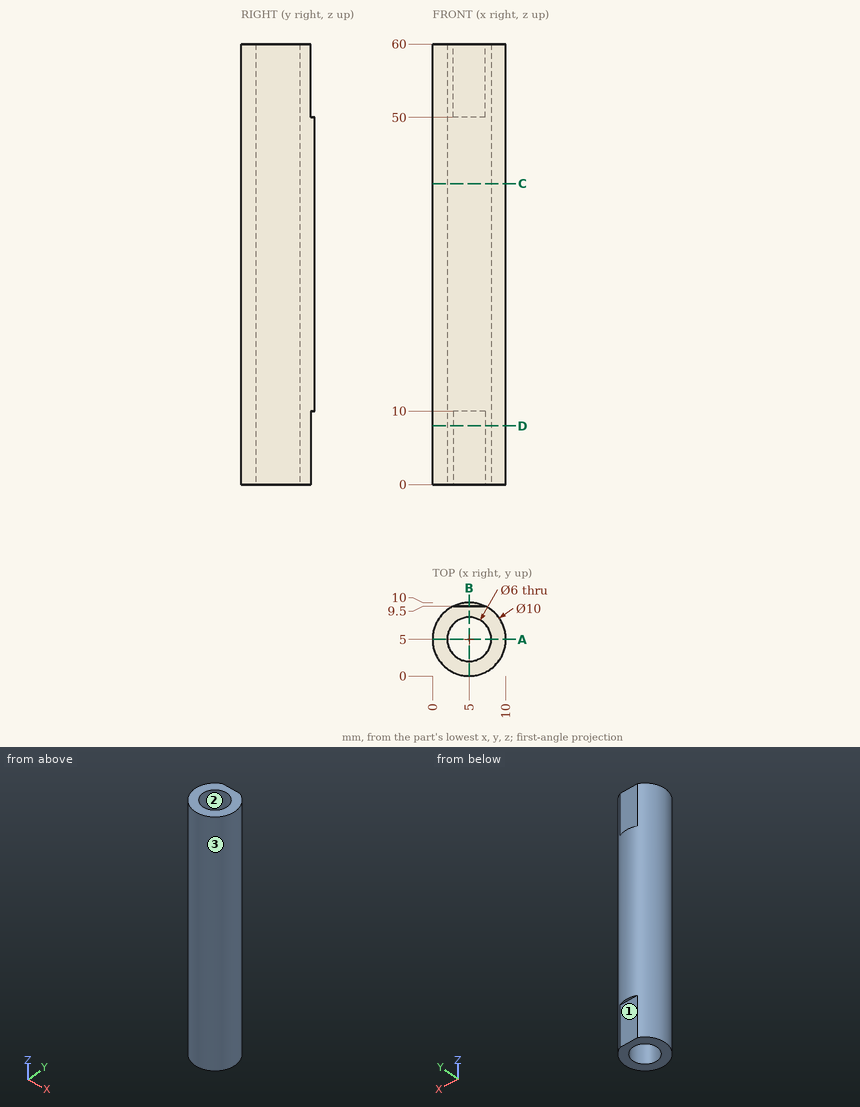
Geometry: see drawing. Coordinates: mm, zero at the bounding-box minimum. Give positions to 0.01 mm unless a question says otherwise; leave off trailing zeros. Write each loop counter-clockwise with the first axis right and the second up, starting at its lowest first coordinate (ties: lowest second). Pieces come first, ordered by that corner, then holes. Notation, with made-up numbers: (-13.75, -4.75) - (37.25, -4.75) arc R31 cw to (37.25, 22.25) - close; hole circle Ø4 at (46, 24.5). An arc over 180 degrees is marked (long way). Return JSON: item names as keys, results as strings. Group by question number.
1) Section B-B on x = 5. Return the cut outline in (y, z), plus the area to 3 significant figures.
2) First-contact query: P1, Ø2, axis at x = 4.5, z = 2.5, coming from the +Y side; P2, Ø1, axis at x = 2, z = 39.5, coming from the -Y side; P3, Ø1.5, axis at x = 7, z = 11, coming from the +Y side. Flat tips, straight axial feed; report the tip coordinate or a pass-through.
3) Section A-A on y = 5. Return the cut outline in (x, z).
4) Section C-C on z = 41. Return the cut outline in (x, y).
5) Mould query, pull axis Y, two halves, no side actions, for the marked faces 1, 2 and 3. Classes: released by +Y, released by -Y, zero draft, split by the parting line, or undercut.
6) Section D-D on z = 8. Return the cut outline in (x, y).
7) Line query: line 1 (Y direction, x = 4.75, z = 23.5); line 2 (Y direction, x = 6, z = 15.5); line 3 (X direction, y = 2.25, z = 25). Output: solid intervals per line, ascending.
Filled in:
{
 "1": {"outline": "(0, 0) - (2, 0) - (2, 60) - (0, 60) - close; (8, 0) - (9.5, 0) - (9.5, 10) - (10, 10) - (10, 50) - (9.5, 50) - (9.5, 60) - (8, 60) - close", "area": "230 mm^2"},
 "2": {"P1": "stops at y = 9.5", "P2": "stops at y = 0.67", "P3": "stops at y = 9.84"},
 "3": {"outline": "(0, 0) - (2, 0) - (2, 60) - (0, 60) - close; (8, 0) - (10, 0) - (10, 60) - (8, 60) - close"},
 "4": {"outline": "circle Ø10 at (5, 5); hole circle Ø6 at (5, 5)"},
 "5": {"face 1": "released by +Y", "face 2": "undercut", "face 3": "split by the parting line"},
 "6": {"outline": "(2.82, 9.5) arc R5 ccw (long way) to (7.18, 9.5) - close; hole circle Ø6 at (5, 5)"},
 "7": {"line 1": "y = 0.01 to 2.01, 7.99 to 9.99", "line 2": "y = 0.1 to 2.17, 7.83 to 9.9", "line 3": "x = 0.82 to 3.8, 6.2 to 9.18"}
}
